from build123d import *

# Parameters (mm, degrees)
SKETCH_1_W          = 250
SKETCH_1_H          = 70
EXTRUDE_1_DEPTH     = 8
SKETCH_2_R          = 1.75
CUT_EXTRUDE_1_DEPTH = 8
SKETCH_3_W          = 10
SKETCH_3_H          = 70
EXTRUDE_2_DEPTH     = 50
SKETCH_4_W          = 42
SKETCH_4_H          = 10
EXTRUDE_3_DEPTH     = 62
FILLET_2_R          = 5
SKETCH_6_R          = 8
SKETCH_6_R_2        = 2.5
EXTRUDE_4_DEPTH     = 15
FILLET_3_R          = 5


with BuildPart() as part:
    # 草图1 → 凸台-拉伸1 (new body)
    with BuildSketch(Plane(origin=(0, 0, 0), x_dir=(1, 0, 0), z_dir=(0, 1, 0))):
        with Locations((125, 35)):
            Rectangle(SKETCH_1_W, SKETCH_1_H)
    extrude(amount=EXTRUDE_1_DEPTH)

    # 草图2 → 切除-拉伸1 (cut)
    with BuildSketch(Plane(origin=(0, 8, 0), x_dir=(1, 0, 0), z_dir=(0, 1, 0))):
        with Locations(Location((25, 15, 0), (0, 0, 270))):
            Circle(SKETCH_2_R)
        with Locations(Location((225, 15, 0), (0, 0, 270))):
            Circle(SKETCH_2_R)
    extrude(amount=-CUT_EXTRUDE_1_DEPTH, mode=Mode.SUBTRACT)

    # 草图3 → 凸台-拉伸2 (add)
    with BuildSketch(Plane.XZ):
        with Locations((-5, -35)):
            Rectangle(SKETCH_3_W, SKETCH_3_H)
    extrude(amount=-EXTRUDE_2_DEPTH)

    # 草图4 → 凸台-拉伸3 (add)
    with BuildSketch(Plane.ZY.offset(10)):
        with Locations((-49, 55)):
            Rectangle(SKETCH_4_W, SKETCH_4_H)
    extrude(amount=-EXTRUDE_3_DEPTH)

    # 圆角2
    fillet_2_edges = [part.edges().sort_by_distance(p)[0] for p in [
        (0, 50, -49),
        (0, 8, -35),
    ]]
    fillet(fillet_2_edges, radius=FILLET_2_R)

    # 草图6 → 凸台-拉伸4 (add)
    with BuildSketch(Plane(origin=(0, 8, 0), x_dir=(1, 0, 0), z_dir=(0, 1, 0))):
        with Locations(Location((225, 49, 0), (0, 0, 90))):
            Circle(SKETCH_6_R)
        with Locations(Location((225, 49, 0), (0, 0, 270))):
            Circle(SKETCH_6_R_2, mode=Mode.SUBTRACT)
    extrude(amount=EXTRUDE_4_DEPTH)

    # 圆角3
    fillet_3_edges = [part.edges().sort_by_distance(p)[0] for p in [
        (225, 8, -41),
    ]]
    fillet(fillet_3_edges, radius=FILLET_3_R)


solid = part.part
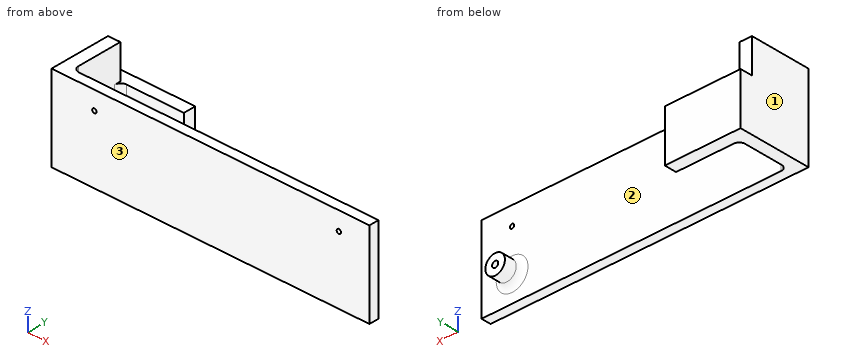
The model under review builds one solid part; all positions refer to its coordinate system, in mm. Face numbers are marked on the shaded views. Coordinates: 2 decimals unless noted, no trailing zeros. Write each loop counter-clockwise with the first axis right and the second up, starting at its lowest first coordinate (ties: lowest second). Pieces come first, ordered by that corner, then holes. Notation, with made-up numbers: M 12.5,16 L 49.5,16 A22 cw 49.5,23 Z; hole C 53.5,-0.5 d7. An arc over 180 degrees is marked long. Put each result on its own line as item: value.
1) Clearance check with flat-ended pins moving along their axes: pin 1 Ø3 at (x, z) = (225, -15) entering from -Y; pin 2 Ø5.5 at (x, z) = (25, -15) entering from +Y; pin 3 Ø6.5 at (x, z) = (225, -49) entering from +Y; pin 4 Ø8 at (y, z) = (56, -43.5) entering from +X. State where each tip first meets the part, or that it passes through.
Computed:
pin 1: passes through
pin 2: stops at y = 8
pin 3: stops at y = 23
pin 4: stops at x = 52
2) Wall thickness on probe 1 along X at (y, z) = (4, -15); probe 2 along X at (y, z) = (20, -49); probe 3 along Z at (x, y) = (225, 4): over which ranges is each line inside the solid? List them lowest first. Write a range as [from, to].
Computed:
probe 1: x = [-10, 23.25], [26.75, 223.25], [226.75, 250]
probe 2: x = [-10, 0], [217, 222.5], [227.5, 233]
probe 3: z = [-70, -16.75], [-13.25, 0]
3) Add section B-B on x = 102. Give the boundary of the cut face in (y, z).
Computed:
outline: M 0,-70 L 8,-70 L 8,0 L 0,0 Z
4) Add section A-A on z = -49. Give the boundary of the cut face in (x, y).
Computed:
outline: M -10,0 L 250,0 L 250,8 L 238,8 A5 cw 233,13 L 233,23 L 227.5,23 L 227.5,8 L 222.5,8 L 222.5,23 L 217,23 L 217,13 A5 cw 212,8 L 5,8 A5 cw 0,13 L 0,45 A5 cw 5,50 L 52,50 L 52,60 L -10,60 Z
5) Add section C-C on z = -25. Give the boundary of the cut face in (x, y), then the cut area to 3 significant figures.
Computed:
outline: M -10,0 L 250,0 L 250,8 L 5,8 A5 cw 0,13 L 0,50 L -10,50 Z
area: 2,510 mm2
6) Draft analysis for pull direction X (two halves, no side actions). For the marked faces 1, 2 and 3, state which applies: released by +X, released by -X, zero draft, split by the parting line, or undercut.
Computed:
face 1: released by -X
face 2: undercut
face 3: zero draft
